Here's how the part is built. I have some questions about the finished solid (model axes, mm). A direction names the side the tool comes from. Coordinates: 2 decimals unless noted, no trailing zeros. Write each loop counter-clockwise with the first axis right and the second up, starting at its lowest first coordinate (ties: lowest second). Pieces come first, ordered by that corner, then holes.
Item 1: If I drill on line 1 (X direction, y = 22.5, z = 68); line 2 (Y direction, x = 73, z = 64); line 3 (Y direction, x = 19, z = 42), over which ranges is the centre line in solid material (lowest first)?
Item 2: If we section it at D-D (y = 71): Please give me the cut outline in (x, z) (3 decimals).
Item 3: For faces 4 (the face through (38, 0, 39)), 5 (the face through (37, -12.113, 92)), 6 (the face through (38, 127, 39)), 7 (the face through (38, 2.54, 49)), 8 (the face through (76.2, 63, 38)), which set-ups out of +Z, -Z, +X, -X, +Y, -Y let a thin tool reach every point of the face, with its end or its side?
Item 4: If we section it at C-C (z = 72): Please give me the cut outline in (x, y).
Item 5: I'm going to push flat-ended pins straight in: pin 1 Ø2 at (x, y) = (57.5, 121.5) entering from -Z (3 decimals); pin 2 Ø2 at (y, z) = (76.5, 26) entering from -X; pin 3 Ø12 at (y, z) = (112.5, 80.5) entering from +X; pin 4 Ø2 at (x, y) = (77, 98) entering from -Z. Where does each tip first touch, or does it pass through?
Item 6: We'd pull the mould along Z, two halves only. Please class faces 1 (the face through (13.06, 61, 95.52)), 2 (the face through (37, 138.811, 91)), 3 (the face through (60, 61, 94.7)): +Z half, -Z half, draft (parallel to the pull), parting line (faces both ways), or undercut.
Item 7: If we section it at B-B (z = 37.5): Please give me the cut outline in (x, y).
Item 8: If we section it at A-A (y = -5): Please give me the cut outline in (x, z) (3 decimals), then the cut area to 3 significant figures.
from build123d import *

# Parameters (mm, degrees)
F0_W          = 76.2
F0_H          = 76.2
F1_DEPTH      = 127
F3_DEPTH      = 14.65342
F3_DEPTH_BACK = 138.81125
F4_T          = -2.54
F6_W          = 29.8130884767
F6_H          = 30.159747228
F6_W_2        = 28.4264292568
F6_H_2        = 48.6897528172
F7_DEPTH      = 25.4


with BuildPart() as f1:
    # F0 (on Front) → F1 (new body)
    with BuildSketch(Plane.XZ):
        with Locations((38.1, 38.1)):
            Rectangle(F0_W, F0_H)
    extrude(amount=-F1_DEPTH)

    # F2 (on Front) → F3 (join, two sides)
    with BuildSketch(Plane.XZ) as f3_sk:
        Polygon((38.1, 114.3), (38.1, 76.2), (76.2, 76.2), (88.9, 76.2), align=None)
        Polygon((-12.7, 76.2), (0, 76.2), (38.1, 76.2), (38.1, 114.3), align=None)
    extrude(amount=F3_DEPTH)
    extrude(f3_sk.sketch, amount=-F3_DEPTH_BACK)

    # F4
    f4_openings = [f1.faces().sort_by_distance(p)[0] for p in [
        (38.1, 63.5, 0),
    ]]
    offset(amount=F4_T, openings=f4_openings, kind=Kind.INTERSECTION)

    # F6 (on Front) → F7 (cut)
    with BuildSketch(Plane.XZ):
        with Locations((53.8429357111, 43.3164620772)):
            Rectangle(F6_W, F6_H)
        with Locations((18.4832299128, 24.3448764086)):
            Rectangle(F6_W_2, F6_H_2)
    extrude(amount=-F7_DEPTH, mode=Mode.SUBTRACT)


solid = f1.part
Answer list:
1. line 1: x = 0 to 2.54, 73.66 to 76.2
1. line 2: y = 0 to 2.54, 124.46 to 127
1. line 3: y = 124.46 to 127
2. outline: (-12.7, 76.2) - (0, 76.2) - (0, 0) - (2.54, 0) - (2.54, 78.74) - (-5.08, 78.74) - (38.1, 111.125) - (81.28, 78.74) - (73.66, 78.74) - (73.66, 0) - (76.2, 0) - (76.2, 76.2) - (88.9, 76.2) - (38.1, 114.3) - close
3. face 4: -Z, +X, -X, -Y
3. face 5: none
3. face 6: -Z, +X, -X, +Y
3. face 7: -Z
3. face 8: -Z, +X, +Y, -Y
4. outline: (0, 0) - (76.2, 0) - (76.2, 127) - (0, 127) - close; hole (2.54, 2.54) - (73.66, 2.54) - (73.66, 124.46) - (2.54, 124.46) - close
5. pin 1: stops at z = 95.825
5. pin 2: stops at x = 0
5. pin 3: stops at x = 88.9
5. pin 4: stops at z = 0
6. face 1: +Z half
6. face 2: draft
6. face 3: undercut
7. outline: (0, 0) - (4.27, 0) - (4.27, 2.54) - (2.54, 2.54) - (2.54, 124.46) - (73.66, 124.46) - (73.66, 2.54) - (68.75, 2.54) - (68.75, 0) - (76.2, 0) - (76.2, 127) - (0, 127) - close; (32.7, 0) - (38.94, 0) - (38.94, 2.54) - (32.7, 2.54) - close
8. outline: (-12.7, 76.2) - (88.9, 76.2) - (38.1, 114.3) - close; hole (-5.08, 78.74) - (81.28, 78.74) - (38.1, 111.125) - close
8. area: 537 mm2
